For this review, use the dimensioned drawing (mm, ordinates from the lowest corner) and the shaded views. A direction names the side the tool comes from. Coordinates: 2 decimals unless noted, no trailing zeros. Loops run counter-clockwise (first coordinate to the right, second up) from the corner with the lowest first, then second, coordinate; pieces in that order, holes last.
1. Take a section at C-C, the plane z = 1.15. Count the separate pieces of the cut face and the enclosed holes in it.
2. To check wall thickness, follow probe 1 along Y at (x, z) = (20.5, 2.5); probe 2 along X at (y, z) = (17.75, 1.6); probe 3 along Y at (x, z) = (19.25, 2.25). State the ranges of each line that lie inside material, in increasing order.
3. Machinability: for the marked faces 1, 2 and 3, which of the approach directions +Z, -Z, +X, -X, +Y, -Y give a long, thin tool a straight path to every point of the face, cutting with its end or side? Answer none if there is none.
4. Take a section at D-D, the plane x = 20.5. State the section outline as (y, z) points.
5. Clearance check with flat-ended pins moving along their axes: P1, Ø3, axis at x = 14.5, y = 2.5, coming from the -Z side; P2, Ø4.5, axis at x = 12, y = 10.5, coming from the +Z side; P3, Ø0.7, axis at x = 1, y = 13.7, coming from the -Z side. State where each tip first meets the part, or that it passes through.
6. Take a section at B-B, the plane y = 13.7. State the section outline as (x, z) points, then the cut area to 3 significant figures.
7. Mouldability with a two-part tool opening along X and no side actions: class the marked faces 4, 5 and 6 as pulls with the +X half, pulls with the -X half, needs draft (parallel to the pull), parting line crosses it, or undercut.
8. Take a section at A-A, the plane x = 5. State the section outline as (y, z) points.
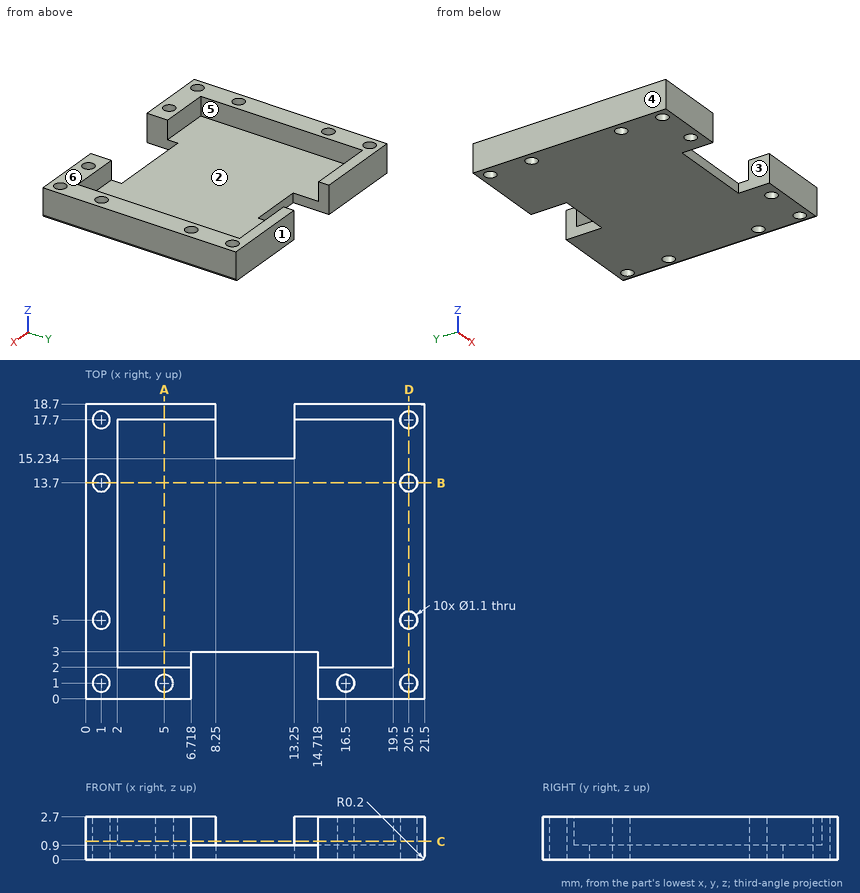
Results list:
1. separate pieces: 2
1. enclosed holes: 10
2. probe 1: y = 0 to 0.45, 1.55 to 4.45, 5.55 to 13.15, 14.25 to 17.15, 18.25 to 18.7
2. probe 2: x = 0 to 0.45, 1.55 to 8.25, 13.25 to 19.95, 21.05 to 21.5
2. probe 3: y = 0 to 2, 17.7 to 18.7
3. face 1: +Z, -Z, +X, -X, +Y
3. face 2: +Z
3. face 3: +Z, -Z, -Y
4. outline: (0, 0) - (0.45, 0) - (0.45, 2.7) - (0, 2.7) - close; (1.55, 0) - (4.45, 0) - (4.45, 2.7) - (1.55, 2.7) - close; (5.55, 0) - (13.15, 0) - (13.15, 2.7) - (5.55, 2.7) - close; (14.25, 0) - (17.15, 0) - (17.15, 2.7) - (14.25, 2.7) - close; (18.25, 0) - (18.7, 0) - (18.7, 2.7) - (18.25, 2.7) - close
5. P1: stops at z = 0
5. P2: stops at z = 0.9
5. P3: passes through
6. outline: (0, 0) - (0.45, 0) - (0.45, 2.7) - (0, 2.7) - close; (1.55, 0) - (19.95, 0) - (19.95, 2.7) - (19.5, 2.7) - (19.5, 0.9) - (2, 0.9) - (2, 2.7) - (1.55, 2.7) - close; (21.05, 0) - (21.3, 0) arc R0.2 ccw to (21.5, 0.2) - (21.5, 2.7) - (21.05, 2.7) - close
6. area: 20.6 mm2
7. face 4: pulls with the -X half
7. face 5: undercut
7. face 6: needs draft
8. outline: (0, 0) - (0.45, 0) - (0.45, 2.7) - (0, 2.7) - close; (1.55, 0) - (18.7, 0) - (18.7, 2.7) - (17.7, 2.7) - (17.7, 0.9) - (2, 0.9) - (2, 2.7) - (1.55, 2.7) - close
